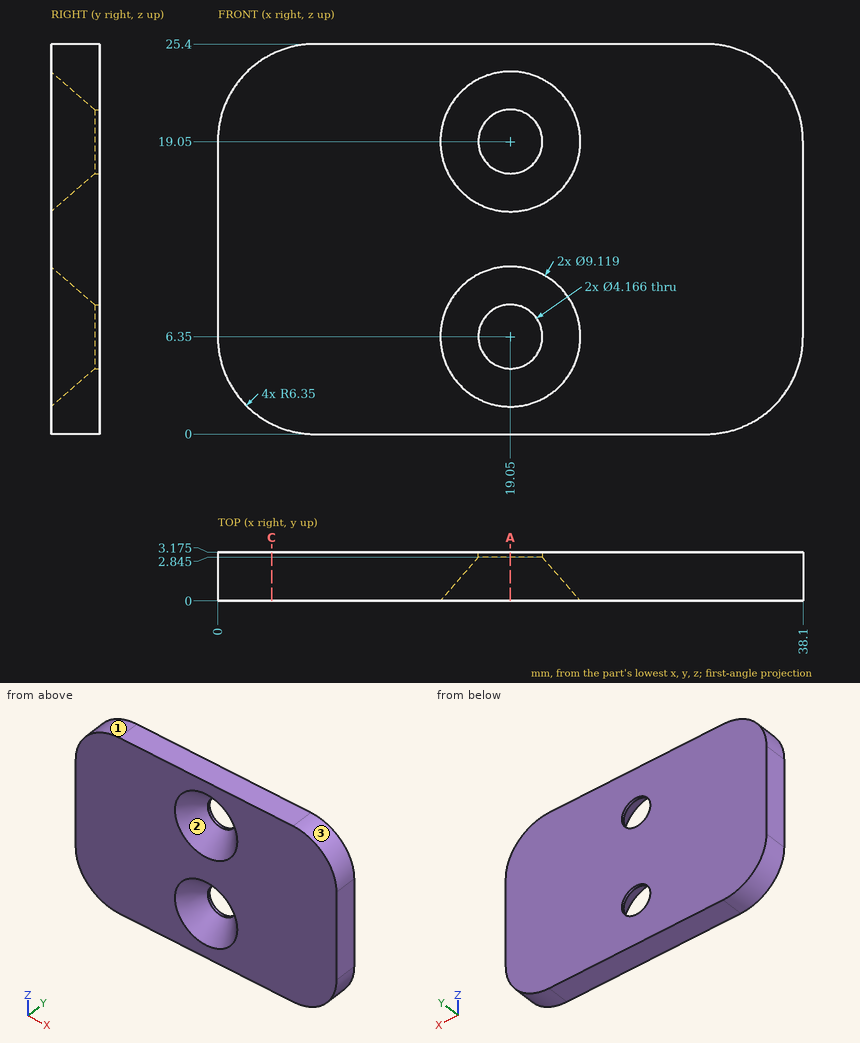
Input: dimensioned drawing with shaded views. Units: mm. Origin: part minimum x, y, z. Give positions to 0.01 mm unless a question says otherwise; leave off trailing zeros. Write each loop counter-clockwise with the first axis right and the second up, starting at its lowest first coordinate (ties: lowest second). Pieces come first, ordered by that corner, then holes.
1. Section query C-C, the plane x = 3.5. Return loops of the section in (y, z) (1 decimal).
2. Pin query (flat end, axial travel): P1, Ø3.5, axis at x = 19.05, z = 6.35, coming from the -Y side; P2, Ø5, axis at x = 24.5, z = 6, coming from the -Y side; P3, Ø1.5, axis at x = 5, y = 2.5, coming from the +Z side. Return the tip coordinate at first contact, or that it passes through.
3. Line query: probe 1 along Z at (x, y) = (19.05, 3); probe 2 along Z at (x, y) = (17.5, 1.25) (1 decimal); probe 3 along X at (y, z) = (0.2, 23) (1 decimal). Output: solid intervals per line, ascending.
4. Draft query along X for the marked faces 1, 2 and 3. Return one class per face: released by +X, released by -X, zero draft, split by the parting line, or undercut.
5. Section query A-A, the plane x = 19.05. Count the separate pieces of the cut face and the enclosed holes in it, then the cut area to 3 significant figures.
Computed:
1. outline: (0, 0.7) - (3.2, 0.7) - (3.2, 24.7) - (0, 24.7) - close
2. P1: passes through
2. P2: stops at y = 0
2. P3: stops at z = 25.37
3. probe 1: z = 0 to 4.27, 8.43 to 16.97, 21.13 to 25.4
3. probe 2: z = 0 to 3.2, 9.5 to 15.9, 22.2 to 25.4
3. probe 3: x = 1.4 to 17.1, 21 to 36.7
4. face 1: released by -X
4. face 2: undercut
4. face 3: released by +X
5. separate pieces: 3
5. enclosed holes: 0
5. area: 40.1 mm2
